```python
from build123d import *

# Parameters (mm, degrees)
SKETCH2_W           = 25.2
SKETCH2_H           = 15
BOSS_EXTRUDE2_DEPTH = 2
SKETCH3_W           = 21.2
SKETCH3_H           = 2
BOSS_EXTRUDE3_DEPTH = 7.8
SKETCH8_W           = 2.35
SKETCH8_H           = 8.163083502
SKETCH8_W_2         = 6.497887862
BOSS_EXTRUDE6_DEPTH = 7.8
SKETCH9_W           = 5
SKETCH9_H           = 8.163083502
SKETCH9_W_2         = 5.002112138
BOSS_EXTRUDE7_DEPTH = 1.3
SKETCH10_W          = 21.2
SKETCH10_H          = 7.8
CUT_EXTRUDE3_DEPTH  = 0.5
SKETCH12_R          = 1
CUT_EXTRUDE4_DEPTH  = 31.920543333
SKETCH13_R          = 2.5
CUT_EXTRUDE5_DEPTH  = 5.634787343


with BuildPart() as part:
    # Sketch2 → Boss-Extrude2 (new body)
    with BuildSketch(Plane.XY):
        with Locations((-12.6, 7.5)):
            Rectangle(SKETCH2_W, SKETCH2_H)
    extrude(amount=BOSS_EXTRUDE2_DEPTH)

    # Sketch3 → Boss-Extrude3 (add)
    with BuildSketch(Plane(origin=(0, 0, 0), x_dir=(-1, 0, 0), z_dir=(0, 0, -1))):
        Polygon((2, 15), (0, 15), (0, 0), (2, 0), (2, 13), align=None)
        with Locations((12.6, 14)):
            Rectangle(SKETCH3_W, SKETCH3_H)
        Polygon((25.2, 15), (23.2, 15), (23.2, 13), (23.2, 0), (25.2, 0), align=None)
    extrude(amount=BOSS_EXTRUDE3_DEPTH)

    # Sketch8 → Boss-Extrude6 (add)
    with BuildSketch(Plane(origin=(0, 0, 0), x_dir=(-1, 0, 0), z_dir=(0, 0, -1))):
        with Locations((3.175, 4.081541751)):
            Rectangle(SKETCH8_W, SKETCH8_H)
        with Locations((12.598943931, 4.081541751)):
            Rectangle(SKETCH8_W_2, SKETCH8_H)
        with Locations((22.025, 4.081541751)):
            Rectangle(SKETCH8_W, SKETCH8_H)
    extrude(amount=BOSS_EXTRUDE6_DEPTH)

    # Sketch9 → Boss-Extrude7 (add)
    with BuildSketch(Plane(origin=(0, 0, 0), x_dir=(-1, 0, 0), z_dir=(0, 0, -1))):
        with Locations((6.85, 4.081541751)):
            Rectangle(SKETCH9_W, SKETCH9_H)
        with Locations((18.348943931, 4.081541751)):
            Rectangle(SKETCH9_W_2, SKETCH9_H)
    extrude(amount=BOSS_EXTRUDE7_DEPTH)

    # Sketch10 → Cut-Extrude3 (cut)
    with BuildSketch(Plane(origin=(0, 15, 0), x_dir=(1, 0, 0), z_dir=(0, 1, 0))):
        with Locations((-12.6, 3.9)):
            Rectangle(SKETCH10_W, SKETCH10_H)
    extrude(amount=-CUT_EXTRUDE3_DEPTH, mode=Mode.SUBTRACT)

    # Sketch12 → Cut-Extrude4 (cut, through all)
    with BuildSketch(Plane.XY.offset(2)):
        with Locations((-12.6, 4)):
            Circle(SKETCH12_R)
    extrude(amount=-CUT_EXTRUDE4_DEPTH, mode=Mode.SUBTRACT)

    # Sketch13 → Cut-Extrude5 (cut)
    with BuildSketch(Plane.XY.offset(2)):
        with Locations((-12.6, 4)):
            Circle(SKETCH13_R)
    extrude(amount=-CUT_EXTRUDE5_DEPTH, mode=Mode.SUBTRACT)


solid = part.part
```
Verification items for the finished model (mm, model axes). A direction names the side the tool comes from. Coordinates: 2 decimals unless noted, no trailing zeros. Write each loop counter-clockwise with the first axis right and the second up, starting at its lowest first coordinate (ties: lowest second). Pieces come first, ordered by that corner, then holes. Notation, with made-up numbers: M 23.25,-38.75 L 74.25,-38.75 A13 ccw 74.25,-18.75 Z; hole C 32,-8 d1. An arc over 180 degrees is marked long. Answer as a JSON object with one key per item and string values. Group by question number.
(1) Gauge pin test, flat ends, axial feed: pin 1 (2.5 mm diameter, centred on x = -6.5, y = 6, fed in from -Z); pin 2 (5 mm diameter, centred on x = -20, z = -1, fed in from -Y); pin 3 (1.6 mm diameter, centred on x = -12.6, y = 4, fed in from -Z). Record the tip position at first contact, or that the pin passes through.
(2) Cross-section at D-D, the plane z = -6.25. Record the cut outline in (x, y).
(3) Cross-section at A-A, the plane z = -3.25. Record the cut outline in (x, y), and give its area (3 significant figures).
(4) Release check for a two-part mould opening along X. For faces 4 (the face through (-25.2, 7, -3)), 5 (the face through (0, 8, -3)), 6 (the face through (-20.85, 4, -5)), 7 (the face through (-12, 5, -7.8)) record: +X half, -X half, draft (parallel to the pull), parting line (faces both ways), or undercut.
(5) Cross-section at B-B, the plane y = 4. Record the cut outline in (x, z).
(6) Material ranges on line 1 (Y direction, x = -12.6, z = -2.45); line 2 (X direction, y = 6.5, z = -7); line 3 (Y direction, x = -12.6, z = 0.8), recorded low to high.
(7) Tool access check on faces 1 (the face through (-15.848, 4, -5)), 2 (the face through (-10.215, 4.751, -0.778)), 3 (the face through (-12, 13, -4)). Record the directions out of +Z, -Z, +X, -X, +Y, -Y that give a thin tool (end or side, any length) a straight path to the whole face; none if there is none.
(8) Cross-section at C-C, the plane x = -12.6. Record the cut outline in (y, z), and give its area (3 significant figures).
Reply:
{
 "1": {"pin 1": "z = -1.3", "pin 2": "y = 0", "pin 3": "through"},
 "2": {"outline": "M -25.2,0 L -20.85,0 L -20.85,8.16 L -23.2,8.16 L -23.2,13 L -2,13 L -2,8.16 L -4.35,8.16 L -4.35,0 L 0,0 L 0,15 L -2,15 L -2,14.5 L -23.2,14.5 L -23.2,15 L -25.2,15 Z; M -15.85,0 L -9.35,0 L -9.35,8.16 L -15.85,8.16 Z; hole C -12.6,4 d2"},
 "3": {"outline": "M -25.2,0 L -20.85,0 L -20.85,8.16 L -23.2,8.16 L -23.2,13 L -2,13 L -2,8.16 L -4.35,8.16 L -4.35,0 L 0,0 L 0,15 L -2,15 L -2,14.5 L -23.2,14.5 L -23.2,15 L -25.2,15 Z; M -15.85,0 L -9.35,0 L -9.35,8.16 L -15.85,8.16 Z; hole C -12.6,4 d5", "area": "164 mm²"},
 "4": {"face 4": "-X half", "face 5": "+X half", "face 6": "undercut", "face 7": "draft"},
 "5": {"outline": "M -25.2,-7.8 L -20.85,-7.8 L -20.85,-1.3 L -15.85,-1.3 L -15.85,-7.8 L -13.6,-7.8 L -13.6,-3.63 L -15.1,-3.63 L -15.1,2 L -25.2,2 Z; M -11.6,-7.8 L -9.35,-7.8 L -9.35,-1.3 L -4.35,-1.3 L -4.35,-7.8 L 0,-7.8 L 0,2 L -10.1,2 L -10.1,-3.63 L -11.6,-3.63 Z"},
 "6": {"line 1": "0 to 1.5, 6.5 to 8.16, 13 to 14.5", "line 2": "-25.2 to -20.85, -15.85 to -9.35, -4.35 to 0", "line 3": "0 to 1.5, 6.5 to 15"},
 "7": {"face 1": "-Z, -Y", "face 2": "+Z", "face 3": "-Z"},
 "8": {"outline": "M 0,-7.8 L 3,-7.8 L 3,-3.63 L 1.5,-3.63 L 1.5,2 L 0,2 Z; M 5,-7.8 L 8.16,-7.8 L 8.16,0 L 13,0 L 13,-7.8 L 14.5,-7.8 L 14.5,0 L 15,0 L 15,2 L 6.5,2 L 6.5,-3.63 L 5,-3.63 Z", "area": "68.9 mm²"}
}
